The model under review builds one solid part; all positions refer to its coordinate system, in mm. Give positions to 0.01 mm unless a question says otherwise; leave off trailing zeros. Loops run counter-clockwise (first coordinate to the right, second up) from the corner with the lowest first, then second, coordinate; pieces in that order, holes last. Notation, with made-up numbers: (38.5, 64) -> (48.5, 64) arc R11 ccw to (48.5, 85) -> close; hole circle Ø2 at (-28.5, 45.25). An arc over 180 degrees is marked (long way). Write each question's results on one line, items separated by ' | '. Start each with the question number.
Q1. Wall thickness on L1, parallel to X at y = 39, z = 1; L2, parallel to X at y = 10.5, z = 1.2; L3, parallel to Y at x = -30, z = 1.25: over which ranges is each line inside the solid? List them lowest first. Write a range as [from, to].
Q2. We need section C-C (z = 1). Write out the cut boundary in (x, y).
Q3. We need section D-D (y = 44.5). Write out the cut boundary in (x, z), plus the area to 3 significant figures.
Q4. We need section A-A (y = 26). Write out the cut boundary in (x, z).
Q5. Insertion check: pin 1 Ø1 at (y, z) = (64.5, 1) entering from +X; pin 2 Ø0.6 at (x, z) = (-99.5, 1.5) entering from +Y; pin 3 Ø0.6 at (y, z) = (63, 1) entering from -X. Each pin has a flat end and moves straight along its axis. Give the tip position at first contact, or say it passes through.
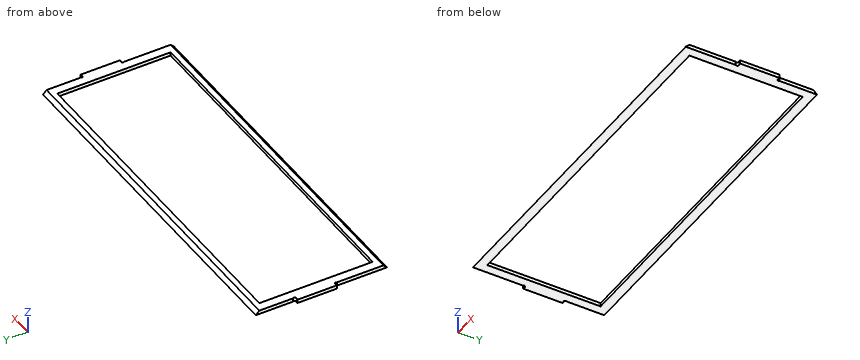
from build123d import *

# Parameters (mm, degrees)
F0_W     = 189.5
F0_H     = 63
F1_DEPTH = 2
F2_SIZE  = 1.99999
F3_SIZE  = 1.99999


# Not quite as in the source:
# - a fillet or chamfer is up to 0.001 mm smaller than in the source, because OpenCascade refuses the exact size


with BuildPart() as f1:
    # F0 (on Top) → F1 (new body)
    with BuildSketch(Plane.XY):
        with BuildLine():
            Line((-99.2, 51), (-100, 51))
            Line((-100, 51), (-100, 29))
            Line((-100, 29), (-99.2, 29))
            ThreePointArc((-99.2, 29), (-98, 29), (-98, 27.8))
            Line((-98, 27.8), (-98, 0))
            Line((-98, 0), (101.5, 0))
            Line((101.5, 0), (101.5, 27.8))
            ThreePointArc((101.5, 27.8), (101.5, 29), (102.7, 29))
            Line((102.7, 29), (103.5, 29))
            Line((103.5, 29), (103.5, 51))
            Line((103.5, 51), (102.7, 51))
            ThreePointArc((102.7, 51), (101.5, 51), (101.5, 52.2))
            Line((101.5, 52.2), (101.5, 73))
            Line((101.5, 73), (-98, 73))
            Line((-98, 73), (-98, 52.2))
            ThreePointArc((-98, 52.2), (-98, 51), (-99.2, 51))
        make_face()
        with Locations((1.75, 36.5)):
            Rectangle(F0_W, F0_H, mode=Mode.SUBTRACT)
    extrude(amount=F1_DEPTH)

    # F2 (size 2 in the source; OpenCascade refuses exactly that, so slightly less here)
    f2_edges = [f1.edges().sort_by_distance(p)[0] for p in [
        (1.75, 0, 2),
    ]]
    chamfer(f2_edges, length=F2_SIZE)

    # F3 (size 2 in the source; OpenCascade refuses exactly that, so slightly less here)
    f3_edges = [f1.edges().sort_by_distance(p)[0] for p in [
        (1.75, 73, 2),
    ]]
    chamfer(f3_edges, length=F3_SIZE)


solid = f1.part
Output:
1) L1: [-100, -93], [96.5, 103.5] | L2: [-98, -93], [96.5, 101.5] | L3: [1.25, 5], [68, 71.75]
2) outline: (-100, 29) -> (-99.2, 29) arc R0.85 cw to (-98, 27.8) -> (-98, 1) -> (101.5, 1) -> (101.5, 27.8) arc R0.85 cw to (102.7, 29) -> (103.5, 29) -> (103.5, 51) -> (102.7, 51) arc R0.85 cw to (101.5, 52.2) -> (101.5, 72) -> (-98, 72) -> (-98, 52.2) arc R0.85 cw to (-99.2, 51) -> (-100, 51) -> close; hole (-93, 5) -> (96.5, 5) -> (96.5, 68) -> (-93, 68) -> close
3) outline: (-100, 0) -> (-93, 0) -> (-93, 2) -> (-100, 2) -> close; (96.5, 0) -> (103.5, 0) -> (103.5, 2) -> (96.5, 2) -> close | area: 28.0 mm2
4) outline: (-98, 0) -> (-93, 0) -> (-93, 2) -> (-98, 2) -> close; (96.5, 0) -> (101.5, 0) -> (101.5, 2) -> (96.5, 2) -> close
5) pin 1: x = 101.5 | pin 2: y = 51 | pin 3: x = -98
